from build123d import *

# Parameters (mm, degrees)
SALIENTE_EXTRUIR2_DEPTH      = 97
REDONDEO2_R                  = 500
SALIENTE_EXTRUIR3_DEPTH      = 26
SALIENTE_EXTRUIR3_DEPTH_BACK = 123
CROQUIS2_R                   = 9.966


with BuildPart() as part:
    # Croquis1 → Saliente-Extruir2 (new body)
    with BuildSketch(Plane.XY):
        with BuildLine():
            Line((0, 40), (100.180824208, 40))
            ThreePointArc((100.180824208, 40), (118.45024357, 35.584102014), (132.685868325, 23.311415808))
            Line((132.685868325, 23.311415808), (277.355906926, 95.588111944))
            Line((277.355906926, 95.588111944), (107.503389255, -39.324038973))
            ThreePointArc((107.503389255, -39.324038973), (103.857673476, -39.830651256), (100.180824208, -40))
            Line((100.180824208, -40), (0, -40))
            ThreePointArc((0, -40), (-40, 0), (0, 40))
        make_face()
    extrude(amount=SALIENTE_EXTRUIR2_DEPTH)

    # Redondeo2
    redondeo2_edges = [part.edges().sort_by_distance(p)[0] for p in [
        (132.685868325, 23.311415808, 48.5),
    ]]
    fillet(redondeo2_edges, radius=REDONDEO2_R)

    # Croquis2 → Saliente-Extruir3 (add, two sides: drawn at the far end of the back side and taken through both)
    with BuildSketch(Plane(origin=(0, 0, 0), x_dir=(-1, 0, 0), z_dir=(0, 0, -1)).offset(-SALIENTE_EXTRUIR3_DEPTH_BACK)):
        Circle(CROQUIS2_R)
    extrude(amount=SALIENTE_EXTRUIR3_DEPTH + SALIENTE_EXTRUIR3_DEPTH_BACK)


solid = part.part
For this review, take the finished solid that the model builds, in its own axes (mm). A direction names the side the tool comes from. Give positions to 0.01 mm unless a question says otherwise; leave off trailing zeros. Loops run counter-clockwise (first coordinate to the right, second up) from the corner with the lowest first, then second, coordinate; pieces in that order, holes last. Notation, with made-up numbers: M -1.5,-25 L 16.5,-25 A22 ccw 16.5,1 Z; hole C 45.25,48 d11. An arc over 180 degrees is marked long. Put each result on its own line as item: value. Start each with the question number.
(1) Machinability: for faces 1 (the flat face through (0, 0, -26)), 2 (the cylindrical face through (2.16, -9.73, 110.18)), 3 (the cylindrical face through (2.16, -9.73, -12.82)), 4 (the flat face through (24, 40, 48)), which of the approach directions +Z, -Z, +X, -X, +Y, -Y give a long, thin tool a straight path to every point of the face, cutting with its end or side? Answer none if there is none.
(2) Add section B-B, the plane x = 22. Write out the cut boundary in (y, z).
(3) Add section A-A, the plane y = 0. Write out the cut boundary in (x, z).
(4) Wall thickness on L1, parallel to Z at x = 6, y = 33; L2, parallel to Y at x = 98.5, z = 42.5; L3, parallel to X at y = -17.5, z = 18: over which ranges is each line inside the solid? List them lowest first.
(5) Add section C-C, the plane y = -23. Write out the cut boundary in (x, z).
(6) For pin 1 (1.5 mm diameter, centred on x = 199.5, y = 54, fed in from -Z); pin 2 (3 mm diameter, centred on y = -5.5, z = 99, fed in from -X); pin 3 (2 mm diameter, centred on x = 222, z = 0.5, fed in from -Y); pin 4 (5 mm diameter, centred on x = 185, y = 62.5, fed in from +Z), all flat-tipped, find the tip position at first contact; note any pin that passes through.
Result:
1. face 1: -Z, +X, -X, +Y, -Y
1. face 2: +Z
1. face 3: -Z
1. face 4: +Z, -Z, -X, +Y
2. outline: M -40,0 L 40,0 L 40,97 L -40,97 Z
3. outline: M -40,0 L -9.97,0 L -9.97,-26 L 9.97,-26 L 9.97,0 L 157.01,0 L 157.01,97 L 9.97,97 L 9.97,123 L -9.97,123 L -9.97,97 L -40,97 Z
4. L1: z = 0 to 97
4. L2: y = -40 to 42.54
4. L3: x = -35.97 to 134.98
5. outline: M -32.73,0 L 128.06,0 L 128.06,97 L -32.73,97 Z
6. pin 1: stops at z = 0
6. pin 2: stops at x = -9.13
6. pin 3: stops at y = 50.83
6. pin 4: passes through
